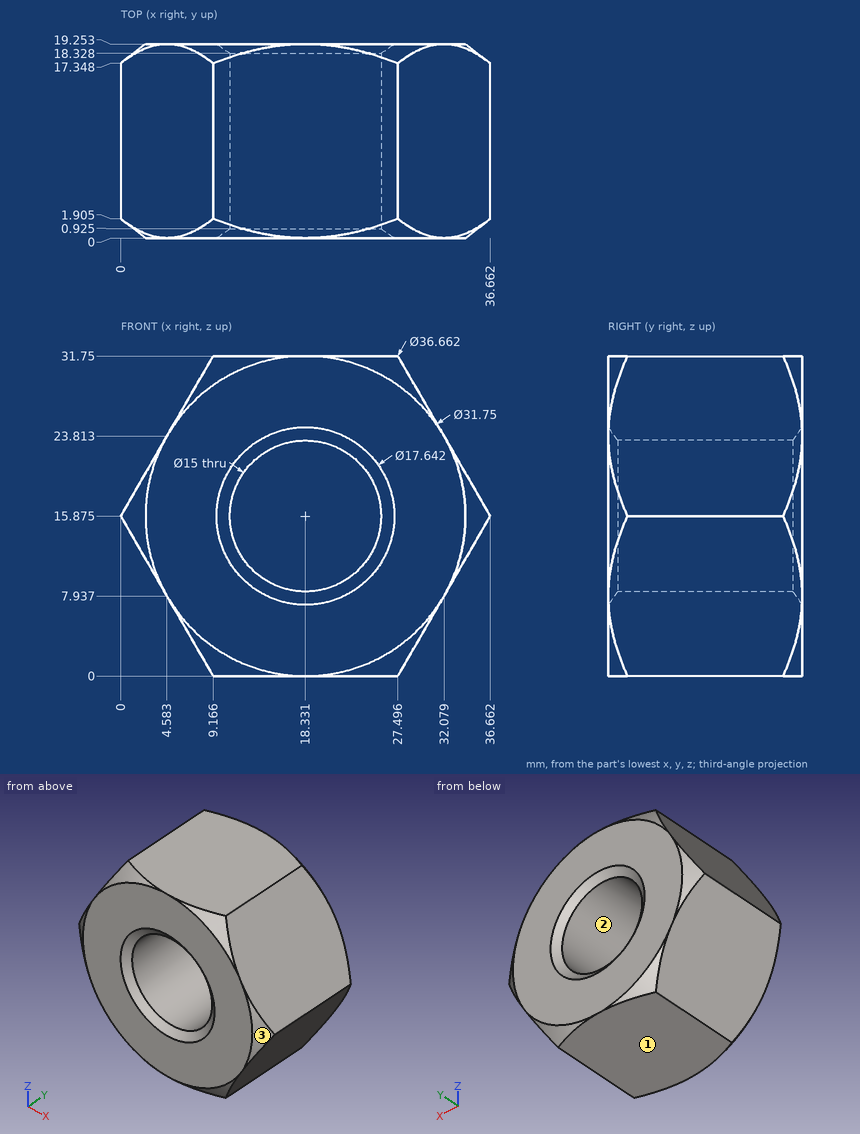
Verification items for this drawing (mm, ordinates from the low corner). Round coordinates to 2 decimals unless told otherwise and drop trailing zeros. Write item = value, one per line. Start each with the question number.
1. Release check for a two-part mould opening along X. For the marked faces 1, 2 and 3 record: pulls with the +X half, pulls with the -X half, needs draft (parallel to the pull), parting line crosses it, or undercut.
2. Gauge pin test, flat ends, axial feed: pin 1 (3 mm diameter, centred on y = 14.5, z = 10.5, fed in from +X) (1 decimal); pin 2 (6 mm diameter, centred on y = 12.5, z = 20.5, fed in from +X); pin 3 (1 mm diameter, centred on y = 12, z = 6, fed in from -X). Record the tip position at first contact, or that the pin passes through.
3. Scan lines: line 1 (X direction, y = 15.25, z = 12) (1 decimal); line 2 (Z direction, x = 22.5, y = 9.75); line 3 (Z direction, x = 16.5, y = 10.25). Record each from-to range of solid material in increasing order. Write a range as [from, to].
Results found:
q1.face_1 = needs draft
q1.face_2 = undercut
q1.face_3 = pulls with the +X half
q2.pin_1 = 34.4
q2.pin_2 = 35.72
q2.pin_3 = 5.41
q3.line_1 = [2.2, 11.9], [24.8, 34.4]
q3.line_2 = [0, 9.64], [22.11, 31.75]
q3.line_3 = [0, 8.6], [23.15, 31.75]
